Autodesk Inventor part; units mm, degrees
ref_plane "YZ Plane" through (0, 0, 0) normal (1, 0, 0) x (0, 1, 0)
ref_plane "XZ Plane" through (0, 0, 0) normal (0, 1, 0) x (-1, 0, 0)
ref_plane "XY Plane" through (0, 0, 0) normal (0, 0, 1) x (1, 0, 0)
sketch "Sketch1" plane through (0, 0, 0) normal (0, 0, 1) x (1, 0, 0)
  line L0 (-68, 115) -> (68, 115)
  line L1 (68, 115) -> (68, -115)
  line L2 (68, -115) -> (-68, -115)
  line L3 (-68, -115) -> (-68, 115)
  line L4 (-68, -115) -> (-38, -115)
  line L5 (-38, -115) -> (-38, -125)
  line L6 (-38, -125) -> (-68, -125)
  line L7 (-68, -125) -> (-68, -115)
  line L8 (38, -115) -> (68, -115)
  line L9 (68, -115) -> (68, -125)
  line L10 (68, -125) -> (38, -125)
  line L11 (38, -125) -> (38, -115)
  point P0 (0, 0)
  point P1 (0, 115)
  point P2 (-68, 0)
  dimension "d0" = 230
  dimension "d1" = 136
  dimension "d49" = 10
  dimension "d50" = 30
extrude "Extrusion1" add sketch "Sketch1" along normal blind 15
sketch "Sketch3" plane through (0, 0, 15) normal (0, 0, 1) x (1, 0, 0)
  circle A0 centre (-60, 103.25) radius 4
  circle A1 centre (60, 103.25) radius 4
  circle A2 centre (60, -113.25) radius 4
  circle A3 centre (-60, -113.25) radius 4
  line L0 (68, 115) -> (-68, 115)
  line L1 (-68, 115) -> (-68, -125)
  line L2 (-38, -115) -> (38, -115)
  line L3 (68, -125) -> (68, 115)
  point P0 (0, 0)
  point P1 (-68, -115)
  dimension "d10" = 11.75
  dimension "d11" = 8
  dimension "d12" = 8
  dimension "d14" = 1.75
  dimension "d60" = 8
extrude "Extrusion3" cut sketch "Sketch3" against normal through all
sketch "Sketch2" plane through (68, -115, 0) normal (1, 0, 0) x (0, 0, -1)
  circle A0 centre (6.5, 200) radius 9.75
  circle A1 centre (6.5, 30) radius 9.75
  line L0 (0, 230) -> (-15, 230)
  circle A2 centre (3.5, 135) radius 9.75
  line L1 (0, -10) -> (0, 230)
  line L2 (0, -10) -> (-15, -10)
  point P0 (0, 115)
  dimension "d6" = 19.5
  dimension "d7" = 30
  dimension "d51" = 6.5
  dimension "d53" = 19.5
  dimension "d54" = 40
  dimension "d55" = 20
  dimension "d56" = 3.5
extrude "Extrusion2" cut sketch "Sketch2" against normal through all
sketch "Sketch4" plane through (0, 0, 15) normal (0, 0, 1) x (1, 0, 0)
  line L0 (-68, 77.7328) -> (68, 77.7328)
  line L1 (68, -77.7328) -> (-68, -77.7328)
  circle A0 centre (60, -113.25) radius 4
  circle A1 centre (60, 103.25) radius 4
  circle A2 centre (-60, -113.25) radius 4
  circle A3 centre (-60, 103.25) radius 4
  line L2 (-38, -115) -> (38, -115)
  line L3 (68, 115) -> (-68, 115)
  line L4 (-14.5, 0) -> (14.5, 0) construction
  line L5 (-68, 62.7328) -> (-29.5, 62.7328)
  line L6 (-29.5, 62.7328) -> (-29.5, -62.7328)
  line L7 (-29.5, -62.7328) -> (-68, -62.7328)
  line L8 (-68, -62.7328) -> (-68, 62.7328)
  line L9 (-68, 115) -> (-68, -125)
  line L10 (38, -115) -> (38, -125)
  line L11 (38, -125) -> (68, -125)
  line L12 (68, -125) -> (68, 115)
  line L13 (-68, -125) -> (-38, -125)
  line L14 (-38, -125) -> (-38, -115)
  line L15 (-68, 115) -> (-68, -125)
  point P0 (0, 0)
  point P1 (-68, -115)
  point P2 (0, 0)
  dimension "d18" = 29
  dimension "d19" = 15
  dimension "d20" = 15
  dimension "d21" = 15
extrude "Extrusion4" cut sketch "Sketch4" against normal through all contours L5 L6 L7 L8
mirror "Mirror1" about plane through (0, 0, 0) normal (1, 0, 0) of "Extrusion4"
sketch "Sketch6" plane through (0, 0, 15) normal (0, 0, 1) x (1, 0, 0)
  circle A0 centre (0, 37.25) radius 2.75
  circle A1 centre (0, 2.75) radius 2.75
  line L0 (-20, -56.5) -> (-20, -71.5)
  line L1 (20, -71.5) -> (-20, -71.5)
  line L2 (20, -71.5) -> (20, -56.5)
  line L3 (20, -56.5) -> (50, -56.5)
  line L4 (50, 56.5) -> (50, -56.5)
  line L5 (50, 56.5) -> (20, 56.5)
  line L6 (20, 56.5) -> (20, 71.5)
  line L7 (-20, 71.5) -> (20, 71.5)
  line L8 (-20, 71.5) -> (-20, 56.5)
  line L9 (-20, 56.5) -> (-50, 56.5)
  line L10 (-50, -56.5) -> (-50, 56.5)
  line L11 (-50, -56.5) -> (-20, -56.5)
  line L12 (29.5, -62.7328) -> (29.5, 62.7328)
  line L13 (68, 115) -> (-68, 115)
  point P0 (0, 0)
  point P1 (29.5, -52.7328)
  point P2 (29.5, 52.7328)
  point P3 (0, 115)
  dimension "d37" = 5.5
  dimension "d39" = 34.5
  dimension "d40" = 77.75
hole "Hole2" at (0, 37.25, 15) at (0, 2.75, 15) direction (0, 0, -1) diameter 5.5 end through all counterbore diameter 10 counterbore depth 5
sketch "Sketch5" plane through (0, 0, 15) normal (0, 0, -1) x (-1, 0, 0)
  circle A0 centre (-60, 103.25) radius 4
  line L0 (-68, -125) -> (-68, 115)
  line L1 (-68, 115) -> (68, 115)
  point P0 (0, 0)
  point P1 (-33.5, 99.7672)
  point P2 (-33.5, 70.2328)
  point P3 (-68, 62.7328)
  dimension "d57" = 34.5
  dimension "d58" = 15.2328
  dimension "d59" = 29.5344
hole "Hole1" at (33.5, 70.2328, 15) at (33.5, 99.7672, 15) direction (0, 0, -1) diameter 5.5 end through all counterbore diameter 10 counterbore depth 5
mirror "Mirror2" about plane through (0, 0, 0) normal (1, 0, 0) of "Hole1"
mirror "Mirror3" about plane through (0, 0, 0) normal (0, 1, 0) of "Hole1", "Mirror2"
fillet "Fillet2" radius 2 10 edges at (-68, 115, 7.5) (-68, 62.7328, 7.5) (-68, -62.7328, 7.5) (-68, -125, 7.5) (-38, -125, 7.5) (-38, -115, 7.5) (38, -115, 7.5) (38, -125, 7.5) (68, -125, 7.5) (68, 115, 7.5)
fillet "Fillet3" radius 10 4 edges at (-29.5, -62.7328, 7.5) (-29.5, 62.7328, 7.5) (29.5, 62.7328, 7.5) (29.5, -62.7328, 7.5)
sketch "Sketch8" plane through (-66, 62.7328, 0) normal (0, -1, 0) x (1, 0, 0)
  circle A0 centre (1.1275, 4.4625) radius 1.7875
  point P0 (66, 0)
hole "Hole4" at (-64.8725, 62.7328, 4.4625) direction (0, 1, 0) diameter 2.459 depth 8.8 tip angle 118
equation "\"d20\" = d19"
equation "\"d21\" = d19"
properties part number "0008-10-006 suport injectomat" material "ABS Plastic"
Design review of the part built by this model. Coordinates are the model's own, in mm. A direction names the side the tool comes from. Round coordinates to 2 decimals unless told otherwise and drop trailing zeros. Order: outer loops, then holes, each group sorted by start corner. A loop starts at its lowest first (then second) coordinate and runs counter-clockwise, first axis right, second up. Notation, with made-up numbers: M -22,-29.75 L -4,-29.75 A31 cw -4,3.25 Z; hole C 22,-6 d2. An arc over 180 degrees is marked long. Put each result on its own line as item: value.
Q1. Consider section C-C (x = 60). State the section outline as (y, z) points, and give its area (3 significant figures).
Reported:
outline: M -125,0 L -117.25,0 L -117.25,15 L -125,15 Z; M -109.25,0 L -92.27,0 A9.75 cw -77.73,0 L -62.73,0 L -62.73,15 L -109.25,15 Z; M 62.73,0 L 77.73,0 A9.75 cw 92.27,0 L 99.25,0 L 99.25,15 L 62.73,15 Z; M 107.25,0 L 115,0 L 115,15 L 107.25,15 Z
area: 1,410 mm²
Q2. Consider section B-B (y = 2.75). State the section outline as (x, z) points.
Reported:
outline: M -29.5,0 L -2.75,0 L -2.75,10 L -5,10 L -5,15 L -29.5,15 Z; M 2.75,0 L 29.5,0 L 29.5,15 L 5,15 L 5,10 L 2.75,10 Z
Q3. Consider section A-A (x = 0). State the section outline as (y, z) points.
Reported:
outline: M -115,0 L -92.27,0 A9.75 cw -77.73,0 L 0,0 L 0,10 L -2.25,10 L -2.25,15 L -115,15 Z; M 5.5,0 L 10.9,0 A9.75 cw 29.1,0 L 34.5,0 L 34.5,10 L 32.25,10 L 32.25,15 L 7.75,15 L 7.75,10 L 5.5,10 Z; M 40,0 L 77.73,0 A9.75 cw 92.27,0 L 115,0 L 115,15 L 42.25,15 L 42.25,10 L 40,10 Z
Q4. Consider section D-D (x = 33.5). State how many separate pieces and enclosed holes the cut face has, and give its area (3 significant figures).
Reported:
separate pieces: 6
enclosed holes: 0
area: 1,140 mm²
Q5. Machinability: for faces 1 (the face through (-33.72, 104.762, 12.465)), 2 (the face through (54, -62.733, 8)), 3 (the face through (33.379, 102.515, 4.93)), which of the approach directions +Z, -Z, +X, -X, +Y, -Y give a long, thin tool a straight path to every point of the face, cutting with its end or side? Answer none if there is none.
Reported:
face 1: +Z
face 2: +Z, -Z, +X
face 3: +Z, -Z
Q6. Insertion check: pin 1 Ø16 at (x, y) = (-33.5, 70.23) entering from +Z; pin 2 Ø3 at (x, y) = (33.5, -99.5) entering from +Z; pin 3 Ø1 at (y, z) = (59, 2) entering from -X; pin 4 Ø8 at (x, y) = (0, 37.25) entering from +Z. Each pin has a flat end and moves straight along its axis. Give the tip position at first contact, or say it passes through.
Reported:
pin 1: z = 15
pin 2: through
pin 3: x = -32.14
pin 4: z = 10
Q7. Draft analysis for pull direction Y (two halves, no side actions). For faces 4 (the face through (-53, -62.733, 8)), 5 (the face through (33.72, -104.762, 12.465)), 6 (the face through (-1, -43, 0)), 7 (the face through (-53, -125, 7)), state which applies: released by +Y, released by -Y, zero draft, split by the parting line, or undercut.
Reported:
face 4: undercut
face 5: undercut
face 6: zero draft
face 7: released by -Y
Q8. To check wall thickness, follow line 1 (Y direction, x = 0, z = 12.65); line 2 (Y direction, x = -60, z = 10.75); line 3 (Y direction, x = -48, z = 12.5). State the ranges of each line that lie inside material, in increasing order.
Reported:
line 1: -115 to -2.25, 7.75 to 32.25, 42.25 to 115
line 2: -125 to -117.25, -109.25 to -62.73, 62.73 to 99.25, 107.25 to 115
line 3: -125 to -62.73, 62.73 to 115
